from build123d import *

# Parameters (mm, degrees)
SKETCH1_R           = 3.175
SKETCH1_R_2         = 9.03605
SKETCH1_W           = 49.9872
SKETCH1_H           = 31.9786
BOSS_EXTRUDE1_DEPTH = 0.79375


with BuildPart() as part:
    # Sketch1 → Boss-Extrude1 (new body)
    with BuildSketch(Plane.XY):
        with BuildLine():
            Line((174.136860842, 46.306847874), (-173.843139158, 46.306847874))
            ThreePointArc((-173.843139158, 46.306847874), (-182.823395279, 42.587103995), (-186.543139158, 33.606847874))
            Line((-186.543139158, 33.606847874), (-186.543139158, -390.573152126))
            ThreePointArc((-186.543139158, -390.573152126), (-182.823395279, -399.553408247), (-173.843139158, -403.273152126))
            Line((-173.843139158, -403.273152126), (174.136860842, -403.273152126))
            ThreePointArc((174.136860842, -403.273152126), (183.117116963, -399.553408247), (186.836860842, -390.573152126))
            Line((186.836860842, -390.573152126), (186.836860842, 33.606847874))
            ThreePointArc((186.836860842, 33.606847874), (183.117116963, 42.587103995), (174.136860842, 46.306847874))
        make_face()
        with Locations((-167.493139158, -388.033152126)):
            Circle(SKETCH1_R, mode=Mode.SUBTRACT)
        with Locations((-167.493139158, -283.258152126)):
            Circle(SKETCH1_R, mode=Mode.SUBTRACT)
        with Locations((-167.493139158, -178.483152126)):
            Circle(SKETCH1_R, mode=Mode.SUBTRACT)
        with Locations((-167.493139158, -73.708152126)):
            Circle(SKETCH1_R, mode=Mode.SUBTRACT)
        with Locations((-167.493139158, 31.066847874)):
            Circle(SKETCH1_R, mode=Mode.SUBTRACT)
        with Locations((-55.733139158, 31.066847874)):
            Circle(SKETCH1_R, mode=Mode.SUBTRACT)
        with Locations((56.026860842, 31.066847874)):
            Circle(SKETCH1_R, mode=Mode.SUBTRACT)
        with Locations((167.786860842, 31.066847874)):
            Circle(SKETCH1_R, mode=Mode.SUBTRACT)
        with Locations((167.786860842, -73.708152126)):
            Circle(SKETCH1_R, mode=Mode.SUBTRACT)
        with Locations((167.786860842, -178.483152126)):
            Circle(SKETCH1_R, mode=Mode.SUBTRACT)
        with Locations((167.786860842, -283.258152126)):
            Circle(SKETCH1_R, mode=Mode.SUBTRACT)
        with Locations((167.786860842, -388.033152126)):
            Circle(SKETCH1_R, mode=Mode.SUBTRACT)
        with Locations((56.026860842, -388.033152126)):
            Circle(SKETCH1_R, mode=Mode.SUBTRACT)
        with Locations((-55.733139158, -388.033152126)):
            Circle(SKETCH1_R, mode=Mode.SUBTRACT)
        with Locations((-76.479037871, -339.905329155)):
            Circle(SKETCH1_R_2, mode=Mode.SUBTRACT)
        with Locations((-76.332177029, -187.094114255)):
            Circle(SKETCH1_R_2, mode=Mode.SUBTRACT)
        with Locations((76.479037871, -187.240975097)):
            Circle(SKETCH1_R_2, mode=Mode.SUBTRACT)
        with Locations((76.332177029, -340.052189997)):
            Circle(SKETCH1_R_2, mode=Mode.SUBTRACT)
        with Locations((13.97, -77.772152126)):
            Circle(SKETCH1_R_2, mode=Mode.SUBTRACT)
        with Locations((-17.78, -77.772152126)):
            Circle(SKETCH1_R_2, mode=Mode.SUBTRACT)
        with Locations((-17.78, 13.286847874)):
            Circle(SKETCH1_R_2, mode=Mode.SUBTRACT)
        with Locations((13.97, 13.286847874)):
            Circle(SKETCH1_R_2, mode=Mode.SUBTRACT)
        with Locations((-123.449539158, -45.882452126)):
            Rectangle(SKETCH1_W, SKETCH1_H, mode=Mode.SUBTRACT)
        Polygon((-114.870386547, -115.040351359), (-114.870386547, -104.031104561), (-139.177931457, -97.926967723), (-148.443139158, -97.926967723), (-148.443139158, -115.040351359), align=None, mode=Mode.SUBTRACT)
        Polygon((-68.280739158, -90.405799119), (-60.65056811, -90.405799119), (-34.707986547, -102.505070352), (-34.707986547, -80.813584087), (-68.280739158, -80.813584087), align=None, mode=Mode.SUBTRACT)
        Polygon((-74.789186547, -115.040351359), (-74.789186547, -104.031104561), (-99.096731457, -97.926967723), (-108.361939158, -97.926967723), (-108.361939158, -115.040351359), align=None, mode=Mode.SUBTRACT)
        Polygon((-74.789186547, -102.505070352), (-74.789186547, -80.813584087), (-108.361939158, -80.813584087), (-108.361939158, -90.405799119), (-100.73176811, -90.405799119), align=None, mode=Mode.SUBTRACT)
        Polygon((-59.015531457, -97.926967723), (-68.280739158, -97.926967723), (-68.280739158, -115.040351359), (-34.707986547, -115.040351359), (-34.707986547, -104.031104561), align=None, mode=Mode.SUBTRACT)
        Polygon((-148.443139158, -80.813584087), (-148.443139158, -90.405799119), (-140.81296811, -90.405799119), (-114.870386547, -102.505070352), (-114.870386547, -80.813584087), align=None, mode=Mode.SUBTRACT)
        with BuildLine():
            Line((56.153860842, -72.392561177), (56.153860842, -63.593743074))
            ThreePointArc((56.153860842, -63.593743074), (37.103860842, -67.993152126), (56.153860842, -72.392561177))
        make_face(mode=Mode.SUBTRACT)
        with BuildLine():
            Line((106.953860842, -72.392561177), (106.953860842, -63.593743074))
            ThreePointArc((106.953860842, -63.593743074), (87.903860842, -67.993152126), (106.953860842, -72.392561177))
        make_face(mode=Mode.SUBTRACT)
        with BuildLine():
            Line((142.513860842, -72.392561177), (142.513860842, -63.593743074))
            ThreePointArc((142.513860842, -63.593743074), (123.463860842, -67.993152126), (142.513860842, -72.392561177))
        make_face(mode=Mode.SUBTRACT)
        with BuildLine():
            Line((130.372660842, -33.13560912), (130.372660842, -26.650695131))
            ThreePointArc((130.372660842, -26.650695131), (115.589860842, -29.893152126), (130.372660842, -33.13560912))
        make_face(mode=Mode.SUBTRACT)
        with BuildLine():
            Line((104.972660842, -33.13560912), (104.972660842, -26.650695131))
            ThreePointArc((104.972660842, -26.650695131), (90.189860842, -29.893152126), (104.972660842, -33.13560912))
        make_face(mode=Mode.SUBTRACT)
        with BuildLine():
            Line((79.572660842, -33.13560912), (79.572660842, -26.650695131))
            ThreePointArc((79.572660842, -26.650695131), (64.789860842, -29.893152126), (79.572660842, -33.13560912))
        make_face(mode=Mode.SUBTRACT)
        with BuildLine():
            Line((54.172660842, -33.13560912), (54.172660842, -26.650695131))
            ThreePointArc((54.172660842, -26.650695131), (39.389860842, -29.893152126), (54.172660842, -33.13560912))
        make_face(mode=Mode.SUBTRACT)
    extrude(amount=BOSS_EXTRUDE1_DEPTH)


solid = part.part
Model file for the job. Use its own axes, mm. A direction names the side the tool comes from. Coordinates: 2 decimals unless noted, no trailing zeros. Order: outer loops, then holes, each group sorted by start corner. A loop starts at its lowest first (then second) coordinate and runs counter-clockwise, first axis right, second up. Notation, with made-up numbers: M -37.75,28.25 L -12.75,28.25 A17 ccw -12.75,38.25 Z; hole C 25.5,61.5 d7. An arc over 180 degrees is marked long. Return JSON: item names as keys, results as strings.
1. Drill centre lines: probe 1 along Y at (x, z) = (-43.5, 0.3); probe 2 along Y at (x, z) = (-116, 0.15); probe 3 along X at (y, z) = (-47.5, 0.6). Where is each one in solid material? Low to high.
Ans:
{"probe 1": "-403.27 to -115.04, -101.82 to -98.4, -80.81 to 46.31", "probe 2": "-403.27 to -115.04, -103.75 to -101.98, -80.81 to -61.87, -29.89 to 46.31", "probe 3": "-186.54 to -148.44, -98.46 to 186.84"}
2. Pull direction X, two halves, no side cores. Call faces 3 (the face through (-182.922, -399.454, 0.391)), 4 (the face through (183.02, -399.65, 0.39)), 5 (the face through (64.795, -29.599, 0.391)): +X half, -X half, draft (parallel to the pull), parting line (faces both ways), or undercut.
Ans:
{"face 3": "-X half", "face 4": "+X half", "face 5": "undercut"}
3. Saw through at C-C (z = 0.15). Give the number of separate pieces and of enclosed holes in the cut face, and give its area (3 significant figures).
Ans:
{"separate pieces": "1", "enclosed holes": "36", "area": "159,000 mm^2"}
4. Saw through at A-A (x = -17.78). Give the cut face in (y, z), and give its area (3 significant figures).
Ans:
{"outline": "M -403.27,0 L -86.81,0 L -86.81,0.79 L -403.27,0.79 Z; M -68.74,0 L 4.25,0 L 4.25,0.79 L -68.74,0.79 Z; M 22.32,0 L 46.31,0 L 46.31,0.79 L 22.32,0.79 Z", "area": "328 mm^2"}
5. Saw through at B-B (x = 136.5). Give the cut face in (y, z).
Ans:
{"outline": "M -403.27,0 L -77.57,0 L -77.57,0.79 L -403.27,0.79 Z; M -58.42,0 L 46.31,0 L 46.31,0.79 L -58.42,0.79 Z"}
6. Tool access for faces 1 (the face through (-2, -175, 0.794)), 2 (the face through (-128.023, -96.371, 0.391)): list every direction of +Z, -Z, +X, -X, +Y, -Y with a clear straight run to the whole face (end or side of a thin tool).
Ans:
{"face 1": "+Z, +X, -X, +Y, -Y", "face 2": "+Z, -Z"}
